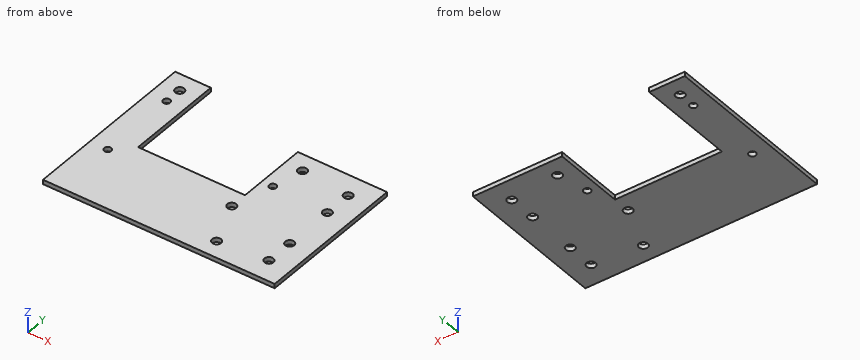
Autodesk Inventor part; units mm, degrees
ref_plane "YZ Plane" through (0, 0, 0) normal (1, 0, 0) x (0, 1, 0)
ref_plane "XZ Plane" through (0, 0, 0) normal (0, 1, 0) x (-1, 0, 0)
ref_plane "XY Plane" through (0, 0, 0) normal (0, 0, 1) x (1, 0, 0)
sketch "Sketch1" plane through (0, 0, 0) normal (0, 0, 1) x (1, 0, 0)
  line L0 (106.0233, -22.2944) -> (-20.9767, -22.2944)
  line L1 (-20.9767, -22.2944) -> (-20.9767, 104.7056)
  line L2 (4.4233, 104.7056) -> (4.4233, 34.8556)
  line L3 (4.4233, 34.8556) -> (80.6233, 34.8556)
  line L4 (-20.9767, 104.7056) -> (4.4233, 104.7056)
  line L5 (106.0233, -22.2944) -> (106.0233, 85.6556)
  line L6 (106.0233, 85.6556) -> (80.6233, 85.6556)
  line L7 (80.6233, 85.6556) -> (80.6233, 34.8556)
  line L8 (106.0233, 85.6556) -> (144.1233, 85.6556)
  line L9 (144.1233, 85.6556) -> (144.1233, -22.2944)
  line L10 (144.1233, -22.2944) -> (106.0233, -22.2944)
  point P0 (0, 0)
  point P1 (-8.2767, 79.4563)
  point P2 (-8.2767, 22.6873)
  point P3 (88.3779, 51.0718)
  point P4 (93.3233, 72.9556)
  point P5 (-8.2767, 92.0056)
  point P6 (80.6233, 22.1556)
  point P7 (93.3233, -9.5944)
  point P8 (128.2483, 13.5704)
  point P9 (128.2483, -6.4194)
  point P10 (128.2483, 69.7552)
  point P11 (128.2483, 49.7654)
  dimension "d0" = 127
  dimension "d5" = 56.769
  dimension "d6" = 96.6546
  dimension "d7" = 12.7
  dimension "d8" = 25.4
  dimension "d9" = 76.2
  dimension "d12" = 107.95
  dimension "d13" = 25.4
  dimension "d14" = 50.8
  dimension "d22" = 28.3845
  dimension "d23" = 127
  dimension "d24" = 25.4
  dimension "d25" = 12.7
  dimension "d26" = 12.7
  dimension "d27" = 44.45
  dimension "d29" = 12.7
  dimension "d30" = 12.7
  dimension "d38" = 12.7
  dimension "d39" = 12.7
  dimension "d40" = 38.1
  dimension "d41" = 107.95
  dimension "d42" = 19.9898
  dimension "d43" = 15.875
  dimension "d53" = 15.875
  dimension "d54" = 15.875
  dimension "d55" = 15.875
  dimension "d56" = 15.875
  dimension "d57" = 15.9004
  dimension "d58" = 19.9898
extrude "Extrusion1" add sketch "Sketch1" against normal blind 3.175 contours L0 L1 L4 L2 L3 L7 L6 L5
hole "Hole1" at (-8.2767, 79.4563, 0) at (-8.2767, 22.6873, 0) at (88.3779, 51.0718, 0) direction (0, 0, -1) diameter 5.0038 depth 25.4 tip angle 118
hole "Hole2" at (93.3233, 72.9556, 0) at (-8.2767, 92.0056, 0) at (80.6233, 22.1556, 0) at (93.3233, -9.5944, 0) direction (0, 0, -1) diameter 6.35 depth 25.4 tip angle 118
extrude "Extrusion2" add sketch "Sketch1" against normal blind 3.175 contours L5 L8 L9 L10
hole "Hole3" at (128.2483, 13.5704, 0) at (128.2483, -6.4194, 0) at (128.2483, 69.7552, 0) at (128.2483, 49.7654, 0) direction (0, 0, -1) diameter 6.35 depth 25.4 tip angle 118
properties part number "AS5-8-5-001"
Can you work these out from the model? Positions are in its coordinate system, mm. Round coordinates to 2 decimals unless told otherwise and drop trailing zeros. Loops run counter-clockwise (first coordinate to the right, second up) from the corner with the lowest first, then second, coordinate; pieces in that order, holes last. Notation, with made-up numbers: M -21,60 L 27,60 A17 ccw 27,78 Z; hole C -38.5,-1.5 d11. An arc over 180 degrees is marked long. Write item = value, one per line. Start each with the question number.
(1) Suppose I cut it at A-A on y = 62. Write out the boundary of the cut face in (x, z) (3 decimals), plus the area to 3 significant figures.
(2) Suppose I cut it at B-B on z = -2.3. Give the number of separate pieces and of enclosed holes in the cut face, plus the area to 3 significant figures.
(3) I need wall thicknesses on line 1 along Y through (x, z) = (93, -2.9); line 2 along Y through (x, z) = (96, -2.05); line 3 along X through (y, z) = (49, -0.5). Which ranges of each line are inside material? Lowest first, please.
(4) Suppose I cut it at C-C on y = 22.5. Write out the boundary of the cut face in (x, z) (3 decimals).
(5) Suppose I cut it at D-D on x = 21.5. Write out the boundary of the cut face in (y, z) (3 decimals).
Answer block:
q1.outline = M -20.977,-3.175 L 4.423,-3.175 L 4.423,0 L -20.977,0 Z; M 80.623,-3.175 L 144.123,-3.175 L 144.123,0 L 80.623,0 Z
q1.area = 282 mm²
q2.separate_pieces = 1
q2.enclosed_holes = 11
q2.area = 14,100 mm²
q3.line_1 = -22.29 to -12.75, -6.44 to 69.8, 76.11 to 85.66
q3.line_2 = -22.29 to -11.3, -7.89 to 71.25, 74.66 to 85.66
q3.line_3 = -20.98 to 4.42, 80.62 to 86.98, 89.78 to 125.17, 131.33 to 144.12
q4.outline = M -20.977,-3.175 L -10.772,-3.175 L -10.772,0 L -20.977,0 Z; M -5.782,-3.175 L 77.467,-3.175 L 77.467,0 L -5.782,0 Z; M 83.78,-3.175 L 144.123,-3.175 L 144.123,0 L 83.78,0 Z
q5.outline = M -22.294,-3.175 L 34.856,-3.175 L 34.856,0 L -22.294,0 Z
